Input: part model. Units: mm. Frame: model coordinates. A direction names the side the tool comes from. Coordinates: 2 decimals unless noted, no trailing zeros. Order: outer loops, then holes, each group sorted by start corner. A loop starts at its lowest first (then second) coordinate and runs counter-clockwise, first axis right, second up. Notation, with made-up numbers: M 33,-38 L 44,-38 A27 cw 44,-5 Z; hole C -17,1.5 d7. An arc over 180 degrees is marked long. Answer in a Markdown table with one row per item.
from build123d import *

# Parameters (mm, degrees)
F1_DEPTH = 6.35
F2_W     = 25.4
F2_H     = 38.1
F2_H_2   = 25.4
F3_DEPTH = 6.351


with BuildPart() as f1:
    # F0 (on Right) → F1 (new body)
    with BuildSketch(Plane.YZ):
        Polygon((-44.45, 28.575), (-44.45, -28.575), (44.45, -28.575), (44.45, 28.575), (44.45, 36.352742), align=None)
    extrude(amount=F1_DEPTH)

    # F2 (on Right) → F3 (cut, through all)
    with BuildSketch(Plane.YZ):
        with Locations((-19.05, -9.525)):
            Rectangle(F2_W, F2_H)
        with Locations((19.05, -3.175)):
            Rectangle(F2_W, F2_H_2)
    extrude(amount=F3_DEPTH, mode=Mode.SUBTRACT)


solid = f1.part
1) Cut plane D-D, the plane y = 25. Output: boundary loops of the cut face in (x, z) (3 decimals).
Resolved:
| item | result |
|---|---|
| outline | M 0,-28.575 L 6.35,-28.575 L 6.35,-15.875 L 0,-15.875 Z; M 0,9.525 L 6.35,9.525 L 6.35,34.651 L 0,34.651 Z |
2) Mould query, pull axis Y, two halves, no side actions, for faces 4 (the face through (3.13, 0.62, 32.52)), 5 (the face through (3, 19, -15.875)), 6 (the face through (3, -19, 9.525)), 7 (the face through (0, -1, 4)). Classes: +Y half, -Y half, draft (parallel to the pull), parting line (faces both ways), or undercut.
Resolved:
| item | result |
|---|---|
| face 4 | -Y half |
| face 5 | undercut |
| face 6 | undercut |
| face 7 | draft |
3) Material intervals for probe 1 along Y at (x, z) = (2.25, 8); probe 2 along Y at (x, z) = (4, -22); probe 3 along Z at (x, y) = (1.5, 26.5) (3 decimals), sorted ascending.
Resolved:
| item | result |
|---|---|
| probe 1 | y = -44.45 to -31.75, -6.35 to 6.35, 31.75 to 44.45 |
| probe 2 | y = -44.45 to -31.75, -6.35 to 44.45 |
| probe 3 | z = -28.575 to -15.875, 9.525 to 34.782 |
4) Cut plane A-A, the plane z = -18. Output: boundary loops of the cut face in (x, y), and give its area (3 significant figures).
Resolved:
| item | result |
|---|---|
| outline | M 0,-44.45 L 6.35,-44.45 L 6.35,-31.75 L 0,-31.75 Z; M 0,-6.35 L 6.35,-6.35 L 6.35,44.45 L 0,44.45 Z |
| area | 403 mm2 |
5) Cut plane B-B, the plane x = 4.75. Output: boundary loops of the cut face in (y, z) (3 decimals).
Resolved:
| item | result |
|---|---|
| outline | M -44.45,-28.575 L -31.75,-28.575 L -31.75,9.525 L -6.35,9.525 L -6.35,-28.575 L 44.45,-28.575 L 44.45,36.353 L -44.45,28.575 Z; hole M 6.35,-15.875 L 31.75,-15.875 L 31.75,9.525 L 6.35,9.525 Z |
6) Contact query for flat-ended pins moving along their axis: pin 1 (3 mm diameter, centred on x = 4, y = 17.5, fed in from +Z); pin 2 (4 mm diameter, centred on y = -28.5, z = -20.5, fed in from +X); pin 3 (1 mm diameter, centred on x = 4.5, y = -24.5, fed in from -Z) (3 decimals). Output: stop coordinate, or through.
Resolved:
| item | result |
|---|---|
| pin 1 | stops at z = 34.13 |
| pin 2 | passes through |
| pin 3 | stops at z = 9.525 |
7) Reachability of faces 1 (the face through (3, -6.35, -10)), 2 (the face through (3, 44.45, 3)), 3 (the face through (3, 31.75, -3)) from +Z, -Z, +X, -X, +Y, -Y: full face, straight path, thin tool, end or side. Return the list, or none.
Resolved:
| item | result |
|---|---|
| face 1 | -Z, +X, -X |
| face 2 | +Z, -Z, +X, -X, +Y |
| face 3 | +X, -X |
8) Cut plane C-C, the plane z = -5.5. Output: boundary loops of the cut face in (x, y), and give its area (3 significant figures).
Resolved:
| item | result |
|---|---|
| outline | M 0,-44.45 L 6.35,-44.45 L 6.35,-31.75 L 0,-31.75 Z; M 0,-6.35 L 6.35,-6.35 L 6.35,6.35 L 0,6.35 Z; M 0,31.75 L 6.35,31.75 L 6.35,44.45 L 0,44.45 Z |
| area | 242 mm2 |
